The listing builds one solid part. Answer for the finished solid, in the listing's coordinates (mm). A direction names the side the tool comes from. Round coordinates to 2 decimals unless told otherwise and drop trailing zeros. Order: outer loops, then holes, each group sorted by start corner. A loop starts at its lowest first (then second) coordinate and runs counter-clockwise, first axis right, second up. Notation, with made-up numbers: (29.5, -32.5) - (85.5, -32.5) arc R14 ccw to (85.5, -20.5) - close; hole circle Ø10 at (47, 33). An arc over 180 degrees is marked (long way). One line per item, written item: value. Start each with the question number.
1. Section D-D, the plane x = -17.5 is taken. Give the vertices of the cut face in (y, z).
2. Flat-ended cylindrical pins translate along their axes: P1, Ø4, axis at y = 9, z = -11, coming from the +X side; P2, Ø10, axis at x = -13.5, y = -20.5, coming from the +Z side; P3, Ø6, axis at y = -3, z = -8.5, coming from the +X side; P4, Ø1, axis at x = -7, y = -12.5, coming from the -Z side. Find the tip coordinate at first contact, or state that the pin passes through.
3. Section A-A, the plane y = 0 is taken. Give the vertices of the cut face in (x, z).
4. Section C-C, the plane z = -3 is taken. Give the vertices of the cut face in (x, y), then the cut area to 3 significant figures.
5. For a pull along Y with two mould halves and no side action, classify faces 3 (the cylindrical face through (-14.985, 0.66, -9.86)), 4 (the cylindrical face through (-5.961, -26.846, -2.465)), 5 (the flat face through (-14, -7, -20)) as released by +Y, released by -Y, zero draft, split by the parting line, or undercut.
6. Straight lines are drawn through the part: line 1 (Z direction, x = 23.5, y = -10); line 2 (Y direction, x = 0, z = -8.5); line 3 (Z direction, x = -1.5, y = 28). For each, find the intervals that lie inside material, in ascending order.
7. A tool of negligible diameter and unlimited length cuts with its end or side. For faces 1 (the flat face through (-23, 0, -5)), 2 (the flat face through (12, -12, 0)), from which of +Z, -Z, +X, -X, +Y, -Y can it reach the whole face along a straight path? Write none if from no direction.
Solid Edge part; units mm, degrees
sketch "Sketch1" plane through (0, 0, 0) normal (0, 0, 1) x (1, 0, 0)
  circle A0 centre (0, 0) radius 27.5
extrude "Protrusion1" add sketch "Sketch1" against normal blind 5
sketch "Sketch2" plane through (0, 0, 0) normal (0, 0, 1) x (1, 0, 0)
  circle A0 centre (0, 0) radius 22.5
extrude "ExtrudedProtrusion_4" add sketch "Sketch2" against normal blind 15
sketch "Sketch3" plane through (0, 0, -15) normal (0, 0, -1) x (1, 0, 0)
  circle A0 centre (0, 0) radius 32.5
extrude "ExtrudedProtrusion_6" add sketch "Sketch3" along normal blind 5
sketch "Sketch4" plane through (0, 0, 0) normal (0, 0, 1) x (1, 0, 0)
  circle A0 centre (0, 0) radius 15
extrude "ExtrudedCutout_2" cut sketch "Sketch4" against normal blind 22
Answer list:
1. outline: (-27.39, -20) - (27.39, -20) - (27.39, -15) - (14.14, -15) - (14.14, -5) - (21.21, -5) - (21.21, 0) - (-21.21, 0) - (-21.21, -5) - (-14.14, -5) - (-14.14, -15) - (-27.39, -15) - close
2. P1: stops at x = 21.38
2. P2: stops at z = 0
2. P3: stops at x = 22.5
2. P4: passes through
3. outline: (-32.5, -20) - (-15, -20) - (-15, 0) - (-27.5, 0) - (-27.5, -5) - (-22.5, -5) - (-22.5, -15) - (-32.5, -15) - close; (15, -20) - (32.5, -20) - (32.5, -15) - (22.5, -15) - (22.5, -5) - (27.5, -5) - (27.5, 0) - (15, 0) - close
4. outline: circle Ø55 at (0, 0); hole circle Ø30 at (0, 0)
4. area: 1,670 mm²
5. face 3: undercut
5. face 4: split by the parting line
5. face 5: zero draft
6. line 1: z = -20 to -15, -5 to 0
6. line 2: y = -22.5 to -15, 15 to 22.5
6. line 3: z = -20 to -15
7. face 1: none
7. face 2: +Z, +X, -X, +Y, -Y
